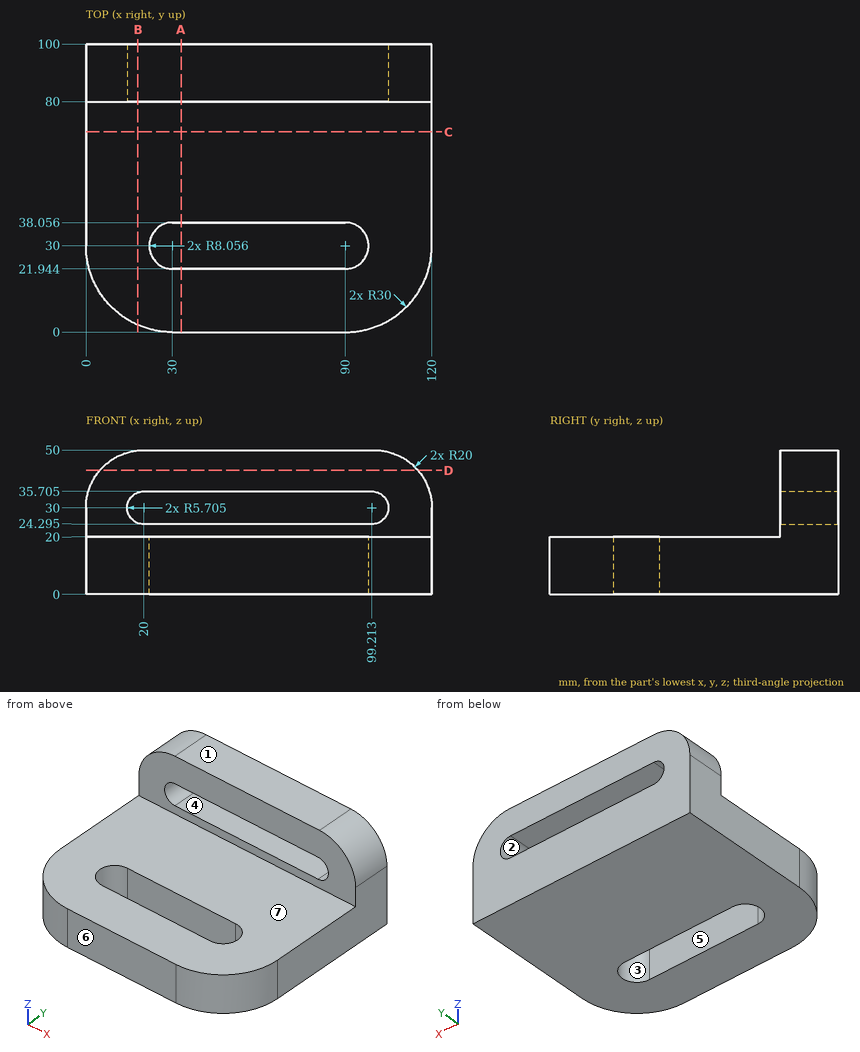
Verification items for this drawing (mm, ordinates from the low corner). A direction names the side the tool comes from. Coordinates: 2 decimals unless noted, no trailing zeros. Order: outer loops, then holes, each group sorted by start corner. A loop starts at its lowest first (then second) coordinate and runs counter-clockwise, first axis right, second up. Notation, with made-up numbers: (88, 3) - (97, 3) arc R20 ccw to (97, 29) - close; hole circle Ø9 at (7.25, 0.25). An arc over 180 degrees is marked (long way). Use one line per item in the form item = value.
1. Section check B-B (x = 18). Record the boundary of the cut face in (y, z), then the cut area to 3 significant figures.
Here are the results:
outline = (2.5, 0) - (100, 0) - (100, 24.66) - (80, 24.66) - (80, 20) - (2.5, 20) - close; (80, 35.34) - (100, 35.34) - (100, 49.9) - (80, 49.9) - close
area = 2,330 mm²
2. Gauge pin test, flat ends, axial feed: pin 1 (4 mm diameter, centred on x = 52, y = 61, fed in from +Z); pin 2 (9 mm diameter, centred on x = 85.5, z = 41, fed in from -Y). Record the tip position at first contact, or that the pin passes through.
Here are the results:
pin_1 = 20
pin_2 = 80
3. Access from +Z, -Z, +X, -X, +Y, -Y to the whole of each face (thin tool, end or side, straight path). Record for the marked faces 4, 5, 6 and 7.
Here are the results:
face_4 = +Y, -Y
face_5 = +Z, -Z
face_6 = +Z, -Z, +X, -X, -Y
face_7 = +Z, +X, -X, -Y
4. Section check C-C (y = 69.5). Record the boundary of the cut face in (x, z), then the cut area to 3 significant figures.
Here are the results:
outline = (0, 0) - (120, 0) - (120, 20) - (0, 20) - close
area = 2,400 mm²
5. Section check A-A (x = 33). Record the boundary of the cut face in (y, z) (1 decimal), then the cut area to 3 significant figures.
Here are the results:
outline = (0, 0) - (21.9, 0) - (21.9, 20) - (0, 20) - close; (38.1, 0) - (100, 0) - (100, 24.3) - (80, 24.3) - (80, 20) - (38.1, 20) - close; (80, 35.7) - (100, 35.7) - (100, 50) - (80, 50) - close
area = 2,050 mm²
6. Scan lines: line 1 (Z direction, x = 29, y = 91) (1 decimal); line 2 (Z direction, x = 12, y = 13.5); line 3 (Y direction, x = 79, z = 9.5). Record each from-to range of solid material in increasing order.
Here are the results:
line_1 = 0 to 24.3, 35.7 to 50
line_2 = 0 to 20
line_3 = 0 to 21.94, 38.06 to 100
7. Section check D-D (z = 43). Record the boundary of the cut face in (x, y).
Here are the results:
outline = (4.8, 80) - (115.2, 80) - (115.2, 100) - (4.8, 100) - close
8. Draft check along Z on the marked faces 1, 2 and 3. Enter one of: pulls with the +Z half, pulls with the -Z half, needs draft (parallel to the pull), parting line crosses it, or undercut.
Here are the results:
face_1 = pulls with the +Z half
face_2 = undercut
face_3 = needs draft
